The listing builds one solid part. Answer for the finished solid, in the listing's coordinates (mm). A direction names the side the tool comes from. Round coordinates to 2 decimals unless told otherwise and drop trailing zeros. Write each loop counter-clockwise with the first axis right and the second up, starting at its lowest first coordinate (ties: lowest second). Pieces come first, ordered by that corner, then holes. Notation, with made-up numbers: (79, 88.5) - (98, 88.5) arc R22 ccw to (98, 97.5) - close; hole circle Ø5 at (-26.75, -39.75). An arc over 180 degrees is marked (long way). Answer in a Markdown table with one row per item.
from build123d import *

# Parameters (mm, degrees)
SKETCH1_R           = 12.7
SKETCH1_R_2         = 7.62
BOSS_EXTRUDE1_DEPTH = 12.7
SKETCH2_R           = 11.43
SKETCH2_R_2         = 8.89
CUT_EXTRUDE1_DEPTH  = 0.254


with BuildPart() as part:
    # Sketch1 → Boss-Extrude1 (new body)
    with BuildSketch(Plane.XY):
        Circle(SKETCH1_R)
        Circle(SKETCH1_R_2, mode=Mode.SUBTRACT)
    extrude(amount=BOSS_EXTRUDE1_DEPTH)

    # Sketch2 → Cut-Extrude1 (cut)
    with BuildSketch(Plane.XY.offset(12.7)):
        Circle(SKETCH2_R)
        Circle(SKETCH2_R_2, mode=Mode.SUBTRACT)
    cut_extrude1 = extrude(amount=-CUT_EXTRUDE1_DEPTH, mode=Mode.SUBTRACT)

    # Mirror1: Cut-Extrude1 across plane
    add(cut_extrude1.mirror(Plane.XY.offset(6.35)), mode=Mode.SUBTRACT)


solid = part.part
(1) Section D-D (y = -9.5) is taken. Give the vertices of the cut face in (x, z), and give its area (3 significant figures).
Checked values:
| item | result |
|---|---|
| outline | (-8.43, 0) - (-6.36, 0) - (-6.36, 0.25) - (6.36, 0.25) - (6.36, 0) - (8.43, 0) - (8.43, 12.7) - (6.36, 12.7) - (6.36, 12.45) - (-6.36, 12.45) - (-6.36, 12.7) - (-8.43, 12.7) - close |
| area | 208 mm2 |
(2) Find the intervals of material crossed by line 1 (Y direction, x = 0, z = 0.15); line 2 (Y direction, x = 0, z = 9.25); line 3 (X direction, y = 4, z = 10.5), in increasing order.
Checked values:
| item | result |
|---|---|
| line 1 | y = -12.7 to -11.43, -8.89 to -7.62, 7.62 to 8.89, 11.43 to 12.7 |
| line 2 | y = -12.7 to -7.62, 7.62 to 12.7 |
| line 3 | x = -12.05 to -6.49, 6.49 to 12.05 |
(3) Flat-ended cylindrical pins translate along their axes: pin 1 (3 mm diameter, centred on y = -9.5, z = 7, fed in from -X); pin 2 (1.5 mm diameter, centred on y = -1, z = 3, fed in from -X); pin 3 (4 mm diameter, centred on y = 4, z = 8.5, fed in from -X). Find the tip coordinate at first contact, or state that the pin passes through.
Checked values:
| item | result |
|---|---|
| pin 1 | stops at x = -9.86 |
| pin 2 | stops at x = -12.7 |
| pin 3 | stops at x = -12.54 |
(4) For a pull along Y with two mould halves and no side action, classify faces 3 (the cylindrical face through (-2.75, -12.4, 6.26)), 4 (the flat face through (6, -7, 0.254)), 5 (the flat face through (7, 4, 0)), 6 (the cylindrical face through (-1.65, -7.44, 6.26)) as pulls with the +Y half, pulls with the -Y half, needs draft (parallel to the pull), parting line crosses it, or undercut.
Checked values:
| item | result |
|---|---|
| face 3 | parting line crosses it |
| face 4 | undercut |
| face 5 | needs draft |
| face 6 | undercut |
(5) For faces 1 (the flat face through (6, -7, 12.446)), 2 (the flat face through (7, 4, 12.7)), determine the directions among +Z, -Z, +X, -X, +Y, -Y from which every point of the face is accessible in a straight line to the end or side of a thin tool.
Checked values:
| item | result |
|---|---|
| face 1 | +Z |
| face 2 | +Z, +X, -X, +Y, -Y |
(6) Section C-C (z = 3) is taken. Give the vertices of the cut face in (x, y), and give its area (3 significant figures).
Checked values:
| item | result |
|---|---|
| outline | circle Ø25.4 at (0, 0); hole circle Ø15.24 at (0, 0) |
| area | 324 mm2 |
(7) Section A-A (y = 0) is taken. Give the vertices of the cut face in (x, z).
Checked values:
| item | result |
|---|---|
| outline | (-12.7, 0) - (-11.43, 0) - (-11.43, 0.25) - (-8.89, 0.25) - (-8.89, 0) - (-7.62, 0) - (-7.62, 12.7) - (-8.89, 12.7) - (-8.89, 12.45) - (-11.43, 12.45) - (-11.43, 12.7) - (-12.7, 12.7) - close; (7.62, 0) - (8.89, 0) - (8.89, 0.25) - (11.43, 0.25) - (11.43, 0) - (12.7, 0) - (12.7, 12.7) - (11.43, 12.7) - (11.43, 12.45) - (8.89, 12.45) - (8.89, 12.7) - (7.62, 12.7) - close |
